```python
from build123d import *

# Parameters (mm, degrees)
SKETCH1_R           = 2
BOSS_EXTRUDE1_DEPTH = 3
CHAMFER1_SIZE       = 0.5


with BuildPart() as part:
    # Sketch1 → Boss-Extrude1 (new body)
    with BuildSketch(Plane.XY):
        with BuildLine():
            Line((-11.019354839, 4), (86.980645161, 4))
            ThreePointArc((86.980645161, 4), (90.980645161, 0), (86.980645161, -4))
            Line((86.980645161, -4), (-11.019354839, -4))
            ThreePointArc((-11.019354839, -4), (-15.019354839, 0), (-11.019354839, 4))
        make_face()
        with Locations((-11.019354839, 0)):
            Circle(SKETCH1_R, mode=Mode.SUBTRACT)
        with Locations((86.980645161, 0)):
            Circle(SKETCH1_R, mode=Mode.SUBTRACT)
    extrude(amount=BOSS_EXTRUDE1_DEPTH)

    # Chamfer1
    chamfer1_edges = [part.edges().sort_by_distance(p)[0] for p in [
        (90.980645161, 0, 3),
        (37.980645161, 4, 3),
        (-15.019354839, 0, 3),
        (37.980645161, 4, 0),
        (90.980645161, 0, 0),
        (37.980645161, -4, 0),
        (-15.019354839, 0, 0),
        (37.980645161, -4, 3),
    ]]
    chamfer(chamfer1_edges, length=CHAMFER1_SIZE)


solid = part.part
```
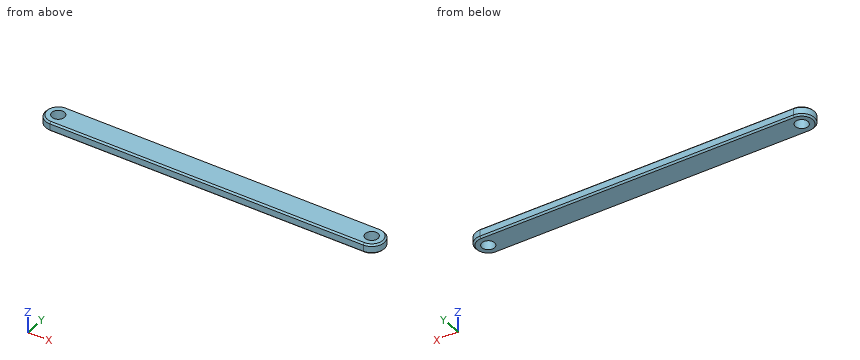
For this review, take the finished solid that the model builds, in its own axes (mm). Round coordinates to 2 decimals unless told otherwise and drop trailing zeros. Order: outer loops, then holes, each group sorted by start corner. A loop starts at its lowest first (then second) coordinate and runs counter-clockwise, first axis right, second up. Notation, with made-up numbers: (-6.5, 30.5) -> (27.5, 30.5) arc R20 cw to (27.5, 67.5) -> close; hole circle Ø6 at (47, 36.25). An arc over 180 degrees is marked (long way). Use a Markdown table: item, result.
Item 1: For pin 1 (1 mm diameter, centred on y = -1.5, z = 0.5, fed in from -X); pin 2 (1 mm diameter, centred on y = 2.5, z = 2, fed in from -X), all flat-tipped, find the tip position at first contact; note any pin that passes through.
Resolved:
| item | result |
|---|---|
| pin 1 | stops at x = -14.89 |
| pin 2 | stops at x = -14.48 |
Item 2: Take a section at B-B (x = -2.5). State the section outline as (y, z) points, plus the area to 3 significant figures.
Resolved:
| item | result |
|---|---|
| outline | (-4, 0.5) -> (-3.5, 0) -> (3.5, 0) -> (4, 0.5) -> (4, 2.5) -> (3.5, 3) -> (-3.5, 3) -> (-4, 2.5) -> close |
| area | 23.5 mm² |
Item 3: For line 1 along X through (y, z) = (-1.5, 1.75); line 2 along X through (y, z) = (0.5, 1.4); line 3 along Y through (x, z) = (23, 2.75), list the stretches that pass through material, from the lowest coordinate up. Write a range as [from, to].
Resolved:
| item | result |
|---|---|
| line 1 | x = [-14.73, -12.34], [-9.7, 85.66], [88.3, 90.69] |
| line 2 | x = [-14.99, -12.96], [-9.08, 85.04], [88.92, 90.95] |
| line 3 | y = [-3.75, 3.75] |
Item 4: Take a section at A-A (y = 0). State the section outline as (x, z) points, plus the area to 4 significant figures.
Resolved:
| item | result |
|---|---|
| outline | (-15.02, 0.5) -> (-14.52, 0) -> (-13.02, 0) -> (-13.02, 3) -> (-14.52, 3) -> (-15.02, 2.5) -> close; (-9.02, 0) -> (84.98, 0) -> (84.98, 3) -> (-9.02, 3) -> close; (88.98, 0) -> (90.48, 0) -> (90.98, 0.5) -> (90.98, 2.5) -> (90.48, 3) -> (88.98, 3) -> close |
| area | 293.5 mm² |
